Here's how the part is built. I have some questions about the finished solid (model axes, mm). A direction names the side the tool comes from. Round coordinates to 2 decimals unless told otherwise and drop trailing zeros. Order: outer loops, then holes, each group sorted by start corner. A loop starts at its lowest first (then second) coordinate and runs counter-clockwise, first axis right, second up. Notation, with made-up numbers: (30, 14.25) -> (83, 14.25) arc R29 ccw to (83, 39.25) -> close; hole circle Ø8 at (-12.5, -20.75). An arc over 180 degrees is marked (long way). Use a Markdown table: item, result. Add a question column.
Autodesk Inventor part; units mm, degrees
ref_plane "Work Plane1" through (64, 103.4423, 140.8327) normal (0, 0.8660254, 0.5) x (1, 0, 0)
ref_plane "Work Plane2" through (32, 26, 47.5) normal (0, 0, 1) x (1, 0, 0)
ref_plane "YZ Plane" through (0, 0, 0) normal (1, 0, 0) x (0, 1, 0)
sketch "Sketch1" plane through (0, 0, 0) normal (0, 1, 0) x (-1, 0, 0)
  line L0 (0, 0) -> (-64, 0)
  line L1 (-64, 0) -> (-64, 140)
  line L2 (-64, 140) -> (0, 140)
  line L3 (0, 140) -> (0, 0)
  dimension "d0" = 140
  dimension "d1" = 64
extrude "Extrusion1" add sketch "Sketch1" along normal blind 19
sketch "Sketch3" plane through (64, 0, 140) normal (1, 0, 0) x (0, 0, -1)
  line L0 (0, 0) -> (-36, 62.3538)
  line L1 (0, 0) -> (72, 0) construction
  line L2 (-36, 62.3538) -> (-19.5455, 71.8538)
  line L3 (-19.5455, 71.8538) -> (21.9393, 0)
  line L4 (0, 0) -> (140, 0)
  line L5 (21.9393, 0) -> (0, 0)
  dimension "d4" = 72
  dimension "d5" = 120
  dimension "d6" = 19
  dimension "d7" = 90
extrude "Extrusion2" add sketch "Sketch3" against normal up to surface (64 mm away)
sketch "Sketch4" plane through (0, 62.3538, 176) normal (0, 0.8660254, 0.5) x (1, 0, 0)
  line L0 (64, 0) -> (0, 0) construction
  line L1 (32, 0) -> (32, 51) construction
  line L2 (32, 0) -> (83, 0) construction
  arc A0 (64, 51) -> (0, 51) centre (32, 51) ccw
  line L3 (0, 51) -> (0, 0)
  line L4 (64, 51) -> (64, 0)
  line L5 (0, 0) -> (64, 0)
  point P0 (0, 121.2436)
  dimension "d10" = 51
  dimension "d11" = 90
  dimension "d12" = 64
extrude "Extrusion3" add sketch "Sketch4" along normal blind 18
sketch "Sketch5" plane through (0, 77.9423, 185) normal (0, 0.8660254, 0.5) x (1, 0, 0)
  line L0 (0, 0) -> (64, 0) construction
  line L1 (32, 0) -> (32, 51) construction
  circle A0 centre (32, 51) radius 9.5
  point P0 (0, 121.2436)
  dimension "d15" = 51
  dimension "d16" = 19
extrude "Extrusion4" cut sketch "Sketch5" against normal up to surface (18 mm away)
sketch "Sketch6" plane through (0, 77.9423, 185) normal (0, 0.8660254, 0.5) x (1, 0, 0)
  circle A0 centre (32, 51) radius 9.5 construction
  circle A1 centre (32, 51) radius 16
  point P0 (0, 121.2436)
  dimension "d19" = 32
extrude "Extrusion5" cut sketch "Sketch6" against normal blind 9
sketch "Sketch9" plane through (0, 77.9423, 185) normal (0, 0.8660254, 0.5) x (1, 0, 0)
  line L0 (0, 0) -> (64, 0) construction
  line L1 (32, 0) -> (32, 83) construction
  arc A0 (64, 51) -> (0, 51) centre (32, 51) ccw construction
  line L2 (32, 0) -> (115, 0) construction
  arc A1 (64, 51) -> (0, 51) centre (32, 51) ccw construction
  line L3 (32, 83) -> (43, 83) construction
  line L4 (32, 83) -> (43, 83) construction
  line L5 (43, 83) -> (21, 83)
  line L6 (21, 83) -> (21, 0)
  line L7 (21, 0) -> (43, 0)
  line L8 (43, 0) -> (43, 83)
  point P0 (0, 121.2436)
  dimension "d22" = 90
  dimension "d23" = 11
  dimension "d24" = 0
  dimension "d25" = 22
  dimension "d26" = 83
extrude "Extrusion6" cut sketch "Sketch9" against normal blind 6
ref_plane "Work Plane1" through (64, 103.4423, 140.8327) normal (0, 0.8660254, 0.5) x (1, 0, 0)
sketch "Sketch10" plane through (64, 103.4423, 140.8327) normal (0, 0.8660254, 0.5) x (1, 0, 0)
  line L0 (-64, -51) -> (-43, -51) construction
  line L1 (-64, -51) -> (-64, -45) construction
  line L2 (-64, 0) -> (-64, -51) construction
  line L3 (-64, -45) -> (0, -45) construction
  line L4 (0, -51) -> (0, 0) construction
  line L5 (-32, -45) -> (-32, -51) construction
  line L6 (-21, -51) -> (-43, -51) construction
  line L7 (-32, -51) -> (-11, -51) construction
  line L8 (-32, -51) -> (-11, -51) construction
  line L9 (-11, -51) -> (-53, -51)
  line L10 (-11, -51) -> (31, -51) construction
  line L11 (-53, -51) -> (-49.5359, -45)
  line L12 (-53, -51) -> (-46.0718, -51) construction
  line L13 (-11, -51) -> (-14.4641, -45)
  line L14 (-49.5359, -45) -> (-14.4641, -45)
  point P0 (-64, 70.2436)
  dimension "d29" = 6
  dimension "d30" = 21
  dimension "d31" = 0
  dimension "d32" = 42
  dimension "d33" = 180
  dimension "d34" = 60
extrude "Extrusion7" cut sketch "Sketch10" against normal up to surface surface through (32, 0, 70) normal (0, 1, 0)
sketch "Sketch11" plane through (0, 19, 0) normal (0, 1, 0) x (1, 0, 0)
  line L0 (64, 0) -> (0, 0) construction
  line L1 (0, 0) -> (0, -140) construction
  line L2 (64, 0) -> (0, 0) construction
  line L3 (0, 0) -> (0, -17) construction
  line L4 (0, -17) -> (64, -17) construction
  line L5 (64, -17) -> (64, 0) construction
  line L6 (64, 0) -> (51, 0) construction
  line L7 (51, 0) -> (51, -17) construction
  line L8 (51, -17) -> (64, -17) construction
  line L9 (64, -17) -> (64, 0) construction
  line L10 (51, -17) -> (13, -17)
  line L11 (13, -17) -> (13, -78)
  line L12 (13, -78) -> (51, -78)
  line L13 (51, -78) -> (51, -17)
  dimension "d39" = 17
  dimension "d40" = 13
  dimension "d41" = 17
  dimension "d42" = 38
  dimension "d43" = 61
extrude "Extrusion8" add sketch "Sketch11" along normal blind 7
sketch "Sketch12" plane through (0, 26, 0) normal (0, 1, 0) x (1, 0, 0)
  line L0 (13, -78) -> (13, -17) construction
  line L1 (13, -47.5) -> (51, -47.5) construction
  line L2 (51, -17) -> (51, -78) construction
  line L3 (13, -17) -> (51, -17) construction
  line L4 (32, -17) -> (32, -78) construction
  line L5 (13, -62) -> (51, -62) construction
  line L6 (51, -62) -> (51, -33) construction
  line L7 (51, -33) -> (13, -33) construction
  line L8 (13, -33) -> (13, -62) construction
  line L9 (13, -62) -> (51, -33) construction
  line L10 (51, -62) -> (13, -33) construction
  line L11 (13, -17) -> (51, -17)
  line L12 (51, -17) -> (51, -33)
  line L13 (51, -33) -> (13, -33)
  line L14 (13, -33) -> (13, -17)
  line L15 (51, -78) -> (13, -78)
  line L16 (13, -62) -> (51, -62)
  line L17 (51, -62) -> (51, -78)
  line L18 (51, -78) -> (13, -78)
  line L19 (13, -78) -> (13, -62)
  point P0 (0, 0)
  point P1 (32, -47.5)
  dimension "d46" = 29
  dimension "d47" = 45
  dimension "d48" = 45
extrude "Extrusion9" add sketch "Sketch12" along normal blind 25 contours L11 L12 L13 L14
ref_plane "Work Plane2" through (32, 26, 47.5) normal (0, 0, 1) x (1, 0, 0)
sketch "Sketch14" plane through (51, 19, 17) normal (0, 0, -1) x (-1, 0, 0)
  line L0 (0, 32) -> (38, 32)
  arc A0 (38, 32) -> (0, 32) centre (19, 32) ccw
  point P0 (51, -19)
extrude "Extrusion10" add sketch "Sketch14" against normal up to surface (16 mm away)
sketch "Sketch15" plane through (51, 19, 17) normal (0, 0, -1) x (-1, 0, 0)
  arc A0 (38, 32) -> (0, 32) centre (19, 32) ccw construction
  line L0 (38, 0) -> (38, 32) construction
  circle A1 centre (19, 32) radius 19
  point P0 (51, -19)
extrude "Extrusion11" add sketch "Sketch15" along normal blind 3
sketch "Sketch16" plane through (32, 51, 14) normal (0, 0, -1) x (-1, 0, 0)
  circle A0 centre (0, 0) radius 9.5
  point P0 (32, -51)
  dimension "d55" = 19
extrude "Extrusion12" cut sketch "Sketch16" against normal up to surface (19 mm away)
mirror "Mirror1" about plane through (32, 26, 47.5) normal (0, 0, 1) of "Extrusion10", "Extrusion11", "Extrusion12", "Extrusion9"
properties part number "1.1"
(1) I'm going to push flat-ended pins straight in: P1, Ø24.5, axis at x = 32, y = 51, coming from the -Z side; P2, Ø10, axis at y = 36, z = 81.5, coming from the -X side; P3, Ø1, axis at x = 31.5, y = 101, coming from the -Z side. Where does each tip first touch, or does it pass through?
(2) I want a section at C-C on x = 57. List the corners of the cut face in (y, z) for me.
(3) I want a section at A-A on z = 64. List the corners of the cut face in (x, y) for me, and give its area (3 significant figures).
(4) I want a section at B-B on y = 14. List the corners of the cut face in (x, z) for me, and give its area (3 significant figures).
(5) On a 3-axis mill with a long thin cutter (end or side, diameter ignored), from which of +Z, -Z, +X, -X, +Y, -Y can I reach the whole of each face in a straight line? I mean faces 1 (the flat face through (32.448, 45.797, 144.502)), 2 (the flat face through (38.9, 92.2, 142.3)), 3 (the flat face through (13, 24, 48)), 4 (the cylindrical face through (39, 44.58, 71.63)), 5 (the flat face through (32, 39, 33)). Say none if no direction works.
(6) I want a section at D-D on z = 167. List the corners of the cut face in (x, y) for me.
(7) Please list where these lines run through material, in increasing order: probe 1 along Z at (x, y) = (24, 61.5); probe 2 along Y at (x, z) = (32, 18.5); probe 3 along Z at (x, y) = (23.5, 35). Write a range as from..to.
(8) If we mould it in two halves opening along Y, with no side actions, what happens to faces 6 (the flat face through (51.29, 39.52, 159.4)), 7 (the flat face through (43, 111, 121)), 8 (the flat face through (24.441, 84.522, 137.603))? For each: pulls with the +Y half, pulls with the -Y half, needs draft (parallel to the pull), parting line crosses it, or undercut.
Output:
| question | item | result |
|---|---|---|
| 1 | P1 | z = 14 |
| 1 | P2 | x = 13 |
| 1 | P3 | z = 108.2 |
| 2 | outline | (0, 0) -> (19, 0) -> (19, 129.03) -> (71.85, 159.55) -> (97.84, 114.53) -> (113.43, 123.53) -> (77.94, 185) -> (62.35, 176) -> (0, 140) -> close |
| 3 | outline | (0, 0) -> (64, 0) -> (64, 19) -> (51, 19) -> (51, 51) arc R19 ccw to (13, 51) -> (13, 19) -> (0, 19) -> close; hole circle Ø19 at (32, 51) |
| 3 | area | 2,720 mm² |
| 4 | outline | (0, 0) -> (64, 0) -> (64, 148.08) -> (53, 148.08) -> (49.54, 141.15) -> (14.46, 141.15) -> (11, 148.08) -> (0, 148.08) -> close |
| 4 | area | 9,210 mm² |
| 5 | face 1 | +X, -X |
| 5 | face 2 | none |
| 5 | face 3 | -Z, -X, +Y |
| 5 | face 4 | -Z |
| 5 | face 5 | +X, -X, +Y |
| 6 | outline | (0, 46.77) -> (11, 46.77) -> (14.46, 58.77) -> (49.54, 58.77) -> (53, 46.77) -> (64, 46.77) -> (64, 88.33) -> (43, 88.33) -> (43, 81.4) -> (21, 81.4) -> (21, 88.33) -> (0, 88.33) -> close |
| 7 | probe 1 | 14..33, 62..81, 153.57..168.58 |
| 7 | probe 2 | 0..41.5, 60.5..70 |
| 7 | probe 3 | 14..33, 62..81, 138.27..153.28 |
| 8 | face 6 | pulls with the -Y half |
| 8 | face 7 | needs draft |
| 8 | face 8 | undercut |
